For this review, take the finished solid that the model builds, in its own axes (mm). A direction names the side the tool comes from. Coordinates: 2 decimals unless noted, no trailing zeros. Loops run counter-clockwise (first coordinate to the right, second up) from the corner with the lowest first, then second, coordinate; pieces in that order, holes last. Notation, with made-up numbers: (83.5, -12.5) -> (106.5, -12.5) arc R13 ccw to (106.5, -8.5) -> close; hole circle Ø3 at (-3, -3). An arc over 180 degrees is marked (long way). Use a Markdown table: item, result.
Autodesk Inventor part; units mm, degrees
ref_plane "YZ Plane" through (0, 0, 0) normal (1, 0, 0) x (0, 1, 0)
ref_plane "XZ Plane" through (0, 0, 0) normal (0, 1, 0) x (-1, 0, 0)
ref_plane "XY Plane" through (0, 0, 0) normal (0, 0, 1) x (1, 0, 0)
sketch "Sketch1" plane through (0, 0, 0) normal (0, 1, 0) x (-1, 0, 0)
  line L0 (0, 0) -> (0, 14.8)
  line L1 (0, 14.8) -> (-2, 14.8)
  line L2 (-2, 14.8) -> (-2, 9.8)
  line L3 (-2, 9.8) -> (-3, 9.8)
  line L4 (-3, 9.8) -> (-3, 2.8)
  line L5 (-3, 2.8) -> (-5, 2.8)
  line L6 (-5, 2.8) -> (-5, 0)
  line L7 (-5, 0) -> (0, 0)
  dimension "d0" = 10
  dimension "d1" = 6
  dimension "d2" = 4
  dimension "d3" = 5
  dimension "d4" = 7
  dimension "d5" = 2.8
revolve "Revolution1" add sketch "Sketch1" angle 360 about axis through (0, 0, 0) along (0, 0, 1)
thread "Thread1"
sketch "Sketch2" plane through (0, 0, 0) normal (0, 0, -1) x (-1, 0, 0)
  line L0 (0, 1.4434) -> (1.25, 0.7217)
  line L1 (1.25, 0.7217) -> (1.25, -0.7217)
  line L2 (1.25, -0.7217) -> (0, -1.4434)
  line L3 (0, -1.4434) -> (-1.25, -0.7217)
  line L4 (-1.25, -0.7217) -> (-1.25, 0.7217)
  line L5 (-1.25, 0.7217) -> (0, 1.4434)
  point P0 (0, 0)
  point P1 (0, 0)
  dimension "d9" = 2.5
extrude "Extrusion1" cut sketch "Sketch2" against normal blind 2
chamfer "Chamfer1" distance 0.43 angle 45 1 edges at (-2, 0, 14.8)
properties part number "DBSY4-7-5" material "Stainless Steel AISI 304"
(1) Mouldability with a two-part tool opening along Y and no side actions: class faces 4 (the face through (1.25, 0, 1)), 5 (the face through (-1.08, 4.88, 1.38)), 6 (the face through (0, 0, 14.8)) as pulls with the +Y half, pulls with the -Y half, needs draft (parallel to the pull), parting line crosses it, or undercut.
Found:
| item | result |
|---|---|
| face 4 | undercut |
| face 5 | parting line crosses it |
| face 6 | needs draft |
(2) Take a section at B-B on y = 4. Write out the cut boundary in (x, z).
Found:
| item | result |
|---|---|
| outline | (-3, 0) -> (3, 0) -> (3, 2.8) -> (-3, 2.8) -> close |
(3) For line 1 along Z through (x, y) = (-1, 2.75); line 2 along Z through (x, y) = (-4, -1.5); line 3 along Y through (x, z) = (0, 6), list the stretches that pass through material, from the lowest coordinate up.
Found:
| item | result |
|---|---|
| line 1 | z = 0 to 9.8 |
| line 2 | z = 0 to 2.8 |
| line 3 | y = -3 to 3 |
(4) Take a section at D-D on y = 2.25. Write out the cut boundary in (x, z), plus the area to 3 significant figures.
Found:
| item | result |
|---|---|
| outline | (-4.47, 0) -> (4.47, 0) -> (4.47, 2.8) -> (1.98, 2.8) -> (1.98, 9.8) -> (-1.98, 9.8) -> (-1.98, 2.8) -> (-4.47, 2.8) -> close |
| area | 52.8 mm^2 |
(5) Take a section at A-A on z = 12. Write out the cut boundary in (x, y), plus the area to 3 significant figures.
Found:
| item | result |
|---|---|
| outline | circle Ø4 at (0, 0) |
| area | 12.6 mm^2 |
(6) For pin 1 Ø4 at (x, z) = (3.5, 12) entering from -Y; pin 2 Ø1.5 at (y, z) = (3, 2) entering from -X; pin 3 Ø2 at (x, y) = (0, -0.5) entering from -Z; pin 4 Ø2 at (y, z) = (3, 8) entering from +X, all flat-tipped, find the tip position at first contact; note any pin that passes through.
Found:
| item | result |
|---|---|
| pin 1 | stops at y = -1.32 |
| pin 2 | stops at x = -4.47 |
| pin 3 | stops at z = 0 |
| pin 4 | stops at x = 2.24 |
(7) For faces 1 (the face through (1.04, -1.04, 0)), 2 (the face through (1, -2, 9.8)), 3 (the face through (0.63, 1.08, 0.99)), list the 3-axis set-ups (+Z, -Z, +X, -X, +Y, -Y) from which the entire face can be reached by the end or side of a thin tool; tool diameter is ignored.
Found:
| item | result |
|---|---|
| face 1 | -Z, +X, -X, +Y, -Y |
| face 2 | +Z |
| face 3 | -Z |
(8) Take a section at C-C on x = -3.75. Write out the cut boundary in (y, z).
Found:
| item | result |
|---|---|
| outline | (-3.31, 0) -> (3.31, 0) -> (3.31, 2.8) -> (-3.31, 2.8) -> close |
